from build123d import *
from build123d.topology import SkipClean

# Parameters (mm, degrees)
SKETCH_1_W                 = 5
SKETCH_1_H                 = 20
EXTRUDE_START              = -5
EXTRUDE_1_DEPTH            = 5
PATTERN_CIRCULAR_3_COUNT   = 3
PATTERN_CIRCULAR_3_ANGLE   = 120
F_3_THE_OTHER_WAY_COUNT    = 3
F_3_THE_OTHER_WAY_ANGLE    = 120
CUT_EXTRUDE_3_DEPTH        = 55.995278612
PATTERN_CIRCULAR_2_COUNT   = 3
PATTERN_CIRCULAR_2_ANGLE   = 120
F_2_THE_OTHER_WAY_COUNT    = 3
F_2_THE_OTHER_WAY_ANGLE    = 120
HOLE_WIZARD_M51_AT_2_COUNT = 2
HOLE_WIZARD_M51_AT_2_PITCH = 15
HOLE_WIZARD_M51_AT_3_COUNT = 2
HOLE_WIZARD_M51_AT_3_PITCH = 25.980762114
HOLE_WIZARD_M51_AT_4_COUNT = 2
HOLE_WIZARD_M51_AT_4_PITCH = 30
HOLE_WIZARD_M51_AT_5_COUNT = 2
HOLE_WIZARD_M51_AT_5_PITCH = 25.980762114
HOLE_WIZARD_M51_AT_6_COUNT = 2
HOLE_WIZARD_M51_AT_6_PITCH = 15
CUT_EXTRUDE_4_DEPTH        = 55.995278612


with BuildPart() as part:
    # Эскиз1 → Повернуть1 (revolve)
    with BuildSketch(Plane.XY, mode=Mode.PRIVATE) as revolve_1_sk:
        with Locations((2.5, 17.5)):
            Rectangle(SKETCH_1_W, SKETCH_1_H)
    revolve(revolve_1_sk.sketch.rotate(Axis((-29.36512031, 0, 0), (1, 0, 0)), 90), axis=Axis((-29.36512031, 0, 0), (1, 0, 0)))

    # Эскиз11 → Бобышка-Вытянуть1 (add)
    with BuildSketch(Plane.ZY.offset(EXTRUDE_START)):
        with BuildLine():
            Line((-5.543277195, 37.296100594), (-10.456537126, 25.434441832))
            ThreePointArc((-10.456537126, 25.434441832), (0, 27.5), (10.456537126, 25.434441832))
            Line((10.456537126, 25.434441832), (5.543277195, 37.296100594))
            ThreePointArc((5.543277195, 37.296100594), (0, 41), (-5.543277195, 37.296100594))
        make_face()
    extrude_1 = extrude(amount=EXTRUDE_1_DEPTH)

    # Круговой массив3: Бобышка-Вытянуть1 ×3 about axis
    pattern_circular_3_axis = Axis((0, 0, 0), (-1, 0, 0))
    for i in range(1, PATTERN_CIRCULAR_3_COUNT):
        add(extrude_1.rotate(pattern_circular_3_axis, i * PATTERN_CIRCULAR_3_ANGLE / (PATTERN_CIRCULAR_3_COUNT - 1)))

    # 3 the other way: Бобышка-Вытянуть1 ×3 about axis
    f_3_the_other_way_axis = Axis((0, 0, 0), (1, 0, 0))
    for i in range(1, F_3_THE_OTHER_WAY_COUNT):
        add(extrude_1.rotate(f_3_the_other_way_axis, i * F_3_THE_OTHER_WAY_ANGLE / (F_3_THE_OTHER_WAY_COUNT - 1)))

    # Эскиз6 → Вырез-Вытянуть3 (cut, symmetric)
    with BuildSketch(Plane.ZY):
        with BuildLine():
            Line((-3.1, 35.5), (-3.1, 34.5))
            ThreePointArc((-3.1, 34.5), (0, 31.4), (3.1, 34.5))
            Line((3.1, 34.5), (3.1, 35.5))
            ThreePointArc((3.1, 35.5), (0, 38.6), (-3.1, 35.5))
        make_face()
    cut_extrude_3 = extrude(amount=CUT_EXTRUDE_3_DEPTH, both=True, mode=Mode.SUBTRACT)

    # Круговой массив2: Вырез-Вытянуть3 ×3 about axis
    pattern_circular_2_axis = Axis((0, 0, 0), (-1, 0, 0))
    for i in range(1, PATTERN_CIRCULAR_2_COUNT):
        add(cut_extrude_3.rotate(pattern_circular_2_axis, i * PATTERN_CIRCULAR_2_ANGLE / (PATTERN_CIRCULAR_2_COUNT - 1)), mode=Mode.SUBTRACT)

    # 2 the other way: Вырез-Вытянуть3 ×3 about axis
    f_2_the_other_way_axis = Axis((0, 0, 0), (1, 0, 0))
    for i in range(1, F_2_THE_OTHER_WAY_COUNT):
        add(cut_extrude_3.rotate(f_2_the_other_way_axis, i * F_2_THE_OTHER_WAY_ANGLE / (F_2_THE_OTHER_WAY_COUNT - 1)), mode=Mode.SUBTRACT)

    # Эскиз10 → Зенковка для винта с потайной головкой и внутренним шестигранником M51 (revolve, cut)
    with BuildSketch(Plane.ZX.offset(15)):
        Polygon((0, 0), (0, 5), (2.6, 5), (2.6, 2.9), (5.5, 0), align=None)
    hole_wizard_m51 = revolve(axis=Axis((-6.35, 15, 0), (1, 0, 0)), mode=Mode.SUBTRACT)

    # Зенковка для винта с потайной головкой и внутренним шестигранником M51 at 2: Зенковка для винта с потайной головкой и внутренним шестигранником M51 ×2
    with Locations(*[Vector(0, -0.4999999999999632, 0.8660254037844599) * (i * HOLE_WIZARD_M51_AT_2_PITCH) for i in range(1, HOLE_WIZARD_M51_AT_2_COUNT)]):
        add(hole_wizard_m51, mode=Mode.SUBTRACT)

    # Зенковка для винта с потайной головкой и внутренним шестигранником M51 at 3: Зенковка для винта с потайной головкой и внутренним шестигранником M51 ×2
    with Locations(*[Vector(0, -0.8660254037844174, 0.5000000000000369) * (i * HOLE_WIZARD_M51_AT_3_PITCH) for i in range(1, HOLE_WIZARD_M51_AT_3_COUNT)]):
        add(hole_wizard_m51, mode=Mode.SUBTRACT)

    # Зенковка для винта с потайной головкой и внутренним шестигранником M51 at 4: Зенковка для винта с потайной головкой и внутренним шестигранником M51 ×2
    with Locations(*[(0, -i * HOLE_WIZARD_M51_AT_4_PITCH, 0) for i in range(1, HOLE_WIZARD_M51_AT_4_COUNT)]):
        add(hole_wizard_m51, mode=Mode.SUBTRACT)

    # Зенковка для винта с потайной головкой и внутренним шестигранником M51 at 5: Зенковка для винта с потайной головкой и внутренним шестигранником M51 ×2
    with Locations(*[Vector(0, -0.8660254037844599, -0.49999999999996314) * (i * HOLE_WIZARD_M51_AT_5_PITCH) for i in range(1, HOLE_WIZARD_M51_AT_5_COUNT)]):
        add(hole_wizard_m51, mode=Mode.SUBTRACT)

    # Зенковка для винта с потайной головкой и внутренним шестигранником M51 at 6: Зенковка для винта с потайной головкой и внутренним шестигранником M51 ×2
    with Locations(*[Vector(0, -0.5000000000000366, -0.8660254037844176) * (i * HOLE_WIZARD_M51_AT_6_PITCH) for i in range(1, HOLE_WIZARD_M51_AT_6_COUNT)]):
        add(hole_wizard_m51, mode=Mode.SUBTRACT)

    # Эскиз12 → Вырез-Вытянуть4 (cut, through all)
    with SkipClean():  # the faces are left unmerged after this step: merging them gives an invalid solid
        with BuildSketch(Plane.ZY):
            with BuildLine():
                Line((10.456537126, 25.434441832), (5.543277195, 37.296100594))
                ThreePointArc((5.543277195, 37.296100594), (0, 41), (-5.543277195, 37.296100594))
                Line((-5.543277195, 37.296100594), (-10.456537126, 25.434441832))
                ThreePointArc((-10.456537126, 25.434441832), (0, 27.5), (10.456537126, 25.434441832))
            make_face()
        extrude(amount=-CUT_EXTRUDE_4_DEPTH, mode=Mode.SUBTRACT)


solid = part.part
Check sheet for the modelled part. Datum: model origin and axes. Units: mm. A direction names the side the tool comes from. Coordinates: 2 decimals unless noted, no trailing zeros. Write each loop counter-clockwise with the first axis right and the second up, starting at its lowest first coordinate (ties: lowest second). Pieces come first, ordered by that corner, then holes. Notation, with made-up numbers: M 87,84.5 L 119,84.5 A14 ccw 119,103.5 Z; hole C 89.5,-25.5 d9. An arc over 180 degrees is marked long. Answer as CSV lines item,"result".
Q1. Mould release check, pull along Z, two halves, no side actions. Record for faces 1 (the face through (2.535, -8.683, -31.108)), 2 (the face through (2.5, 0.1, 27.5)), 3 (the face through (2.54, -22.6, 23.07)), 4 (the face through (2.535, -22.622, -23.252)): released by +Z, released by -Z, zero draft, split by the parting line, or undercut.
Check result:
face 1,"released by -Z"
face 2,"released by +Z"
face 3,"undercut"
face 4,"undercut"
Q2. Material ranges on probe 1 along Y at (x, z) = (3.8, 0); probe 2 along Y at (x, z) = (4.65, 31); probe 3 along Z at (x, y) = (4.4, -15), recorded low to high. Write a range as from..to.
Check result:
probe 1,"-27.5..-17.6, -12.4..-7.5, 7.5..12.4, 17.6..27.5"
probe 2,"-23.46..-20.84, -14.36..-8.54, 8.54..14.36, 20.84..23.46"
probe 3,"-35.77..-32.18, -27.75..-2.6, 2.6..27.75, 32.18..35.77"
Q3. Go/stop test with flat-tipped pins: pin 1 (24 mm diameter, centred on y = 0, z = 0, fed in from -X); pin 2 (1.5 mm diameter, centred on x = 0.5, z = 6.5, fed in from -Y); pin 3 (1 mm diameter, centred on x = 3, y = 13, fed in from -Z). Record where each tip stops, or that it passes through.
Check result:
pin 1,"x = 0"
pin 2,"y = -26.89"
pin 3,"z = -34.8"
Q4. Set-up check for faces 5 (the face through (2.535, 8.683, 31.108)), 6 (the face through (2.54, 22.6, -23.07)), 7 (the face through (2.5, 8.8, -31.2)): record each of +Z, -Z, +X, -X, +Y, -Y from which the full face is reachable in a straight line by a thin tool's end or side.
Check result:
face 5,"+Z, +X, -X"
face 6,"+X, -X, +Y"
face 7,"-Z, +X, -X"
Q5. Cross-section at A-A (x = 4.25). Count the separate pieces of the cut face and the enclosed holes in it, then the cut area to 3 significant figures.
Check result:
separate pieces,"1"
enclosed holes,"11"
area,"2,690 mm^2"
Q6. Cross-section at C-C (z = 20). Record the boundary of the cut face in (x, y), then the cut area to 3 significant figures.
Check result:
outline,"M 0,-22.19 L 5,-22.19 L 5,22.19 L 0,22.19 Z"
area,"222 mm^2"
